The model under review builds one solid part; all positions refer to its coordinate system, in mm. A direction names the side the tool comes from. Coordinates: 2 decimals unless noted, no trailing zeros. Order: outer loops, then holes, each group sorted by start corner. A loop starts at its lowest first (then second) coordinate and runs counter-clockwise, first axis right, second up. Notation, with made-up numbers: M 31.5,55 L 37.5,55 A12 cw 37.5,67 Z; hole C -4,40.5 d10. An arc over 180 degrees is marked long. Answer as CSV lines item,"result". Start each with the question number.
Q1. Consider section B-B on y = 14.5. Write out the cut boundary in (x, z).
Q2. Consider section C-C on z = 1.5. Write out the cut boundary in (x, y), and give its area (3 significant figures).
Q3. Consider section A-A on x = 0. Write out the cut boundary in (y, z), and give its area (3 significant figures).
Q4. Wall thickness on L1, parallel to Y at x = 0, z = 6; L2, parallel to Y at x = -7, z = -17.5; L3, parallel to Z at x = -20, y = 8.5: over which ranges is each line inside the solid? List them lowest first. Write a range as [from, to].
Q5. For P1, Ø13, axis at x = 8, z = -13, coming from the +Y side; P2, Ø5, axis at y = 29.5, z = 4.5, coming from the +X side; P3, Ø1, axis at x = 4, y = 39, coming from the -Z side, all flat-tipped, find the tip position at first contact; note any pin that passes through.
Q6. The part is to be moulded in two halves that separate along X. For faces 3 (the face through (0.559, 46.984, 6.261)), 4 (the face through (-2.86, 7.708, 6.261)), 5 (the face through (0, 34, 0)), 6 (the face through (-25.4, -4, -2)), say which applies: +X half, -X half, draft (parallel to the pull), parting line (faces both ways), or undercut.
Q7. Machinability: for faces 1 (the face through (0, -11, -25.634)), 2 (the face through (0, 0, -13)), which of the approach directions +Z, -Z, +X, -X, +Y, -Y give a long, thin tool a straight path to every point of the face, cutting with its end or side? Answer none if there is none.
Q8. Consider section D-D on x = 11. Write out the cut boundary in (y, z).
from build123d import *

# Parameters (mm, degrees)
F0_W     = 50.8
F0_H     = 43.18
F1_DEPTH = 12.7
F2_R     = 13.194119
F3_DEPTH = 12.701
F4_W     = 50.8
F4_H     = 25.634238
F5_DEPTH = 21.59


with BuildPart() as f1:
    # F0 (on Top) → F1 (new body)
    with BuildSketch(Plane.XY):
        with BuildLine():
            ThreePointArc((25.4, 21.59), (0, 46.99), (-25.4, 21.59))
            Line((-25.4, 21.59), (25.4, 21.59))
        make_face()
        Rectangle(F0_W, F0_H)
    extrude(amount=F1_DEPTH)

    # F2 (on Top) → F3 (cut, through all)
    with BuildSketch(Plane.XY):
        with Locations((0, 20.587881)):
            Circle(F2_R)
    extrude(amount=F3_DEPTH, mode=Mode.SUBTRACT)

    # F4 (on Front) → F5 (join)
    with BuildSketch(Plane.XZ):
        with Locations((0, -12.817119)):
            Rectangle(F4_W, F4_H)
    extrude(amount=F5_DEPTH)


solid = f1.part
Evaluation:
1,outline,"M -25.4,0 L -11.71,0 L -11.71,12.7 L -25.4,12.7 Z; M 11.71,0 L 25.4,0 L 25.4,12.7 L 11.71,12.7 Z"
2,outline,"M -25.4,-21.59 L 25.4,-21.59 L 25.4,21.59 A25.4 ccw -25.4,21.59 Z; hole C 0,20.59 d26.39"
2,area,"2,660 mm²"
3,outline,"M -21.59,-25.63 L 0,-25.63 L 0,0 L 7.39,0 L 7.39,12.7 L -21.59,12.7 Z; M 33.78,0 L 46.99,0 L 46.99,12.7 L 33.78,12.7 Z"
3,area,"1,090 mm²"
4,L1,"y = [-21.59, 7.39], [33.78, 46.99]"
4,L2,"y = [-21.59, 0]"
4,L3,"z = [0, 12.7]"
5,P1,"stops at y = 0"
5,P2,"stops at x = 24.82"
5,P3,"stops at z = 0"
6,face 3,"parting line"
6,face 4,"undercut"
6,face 5,"draft"
6,face 6,"-X half"
7,face 1,"-Z, +X, -X, +Y, -Y"
7,face 2,"-Z, +X, -X, +Y"
8,outline,"M -21.59,-25.63 L 0,-25.63 L 0,0 L 13.3,0 L 13.3,12.7 L -21.59,12.7 Z; M 27.87,0 L 44.48,0 L 44.48,12.7 L 27.87,12.7 Z"
